Autodesk Inventor part; units mm, degrees
ref_plane "YZ Plane" through (0, 0, 0) normal (1, 0, 0) x (0, 1, 0)
ref_plane "XZ Plane" through (0, 0, 0) normal (0, 1, 0) x (-1, 0, 0)
ref_plane "XY Plane" through (0, 0, 0) normal (0, 0, 1) x (1, 0, 0)
sketch "Sketch1" plane through (0, 0, 0) normal (0, 0, 1) x (1, 0, 0)
  circle A0 centre (0, 0) radius 16.5
  circle A1 centre (15.5, 15.5) radius 1.25
  circle A2 centre (15.5, -15.5) radius 1.55
  circle A3 centre (-15.5, -15.5) radius 1.55
  circle A4 centre (-15.5, 15.5) radius 1.55
  line L0 (-21, 21) -> (21, 21)
  line L1 (21, 21) -> (21, -21)
  line L2 (21, -21) -> (-21, -21)
  line L3 (-21, -21) -> (-21, 21)
  line L4 (-21, 21) -> (21, -21) construction
  line L5 (21, 21) -> (-21, -21) construction
  point P0 (0, 0)
  dimension "d0" = 42
  dimension "d1" = 42
extrude "Extrusion1" add sketch "Sketch1" along normal blind 5
equation "\"BendRadius\" = Thickness"
equation "\"BendReliefWidth\" = Thickness"
equation "\"BendReliefDepth\" = 0.5 * Thickness"
equation "\"CornerReliefSize\" = 4 * Thickness"
equation "\"MinimumRemnant\" = 2 * Thickness"
equation "\"TransitionRadius\" = BendRadius"
equation "\"JacobiRadiusSize\" = Thickness"
equation "\"GapSize\" = Thickness"
properties part number "Motor Mount V2.1"
Here's how the part is built. I have some questions about the finished solid (model axes, mm). Round coordinates to 2 decimals unless told otherwise and drop trailing zeros. Order: outer loops, then holes, each group sorted by start corner. A loop starts at its lowest first (then second) coordinate and runs counter-clockwise, first axis right, second up. Notation, with made-up numbers: (-25.75, 17) -> (29.25, 17) arc R22 cw to (29.25, 23) -> close; hole circle Ø1 at (63, 78.25). An arc over 180 degrees is marked (long way). Use CSV: the item, a comma, the result in double quotes.
1. I want a section at D-D on x = 15.5. List the corners of the cut face in (y, z) for me.
Recorded:
outline,"(-21, 0) -> (-17.05, 0) -> (-17.05, 5) -> (-21, 5) -> close; (-13.95, 0) -> (-5.66, 0) -> (-5.66, 5) -> (-13.95, 5) -> close; (5.66, 0) -> (14.25, 0) -> (14.25, 5) -> (5.66, 5) -> close; (16.75, 0) -> (21, 0) -> (21, 5) -> (16.75, 5) -> close"
2. I want a section at A-A on y = 0. List the corners of the cut face in (x, z) for me, and give its area (3 significant figures).
Recorded:
outline,"(-21, 0) -> (-16.5, 0) -> (-16.5, 5) -> (-21, 5) -> close; (16.5, 0) -> (21, 0) -> (21, 5) -> (16.5, 5) -> close"
area,"45.0 mm2"
3. I want a section at C-C on z = 4.5. List the corners of the cut face in (x, y) for me, and give its area (3 significant figures).
Recorded:
outline,"(-21, -21) -> (21, -21) -> (21, 21) -> (-21, 21) -> close; hole circle Ø3.1 at (-15.5, -15.5); hole circle Ø3.1 at (-15.5, 15.5); hole circle Ø33 at (0, 0); hole circle Ø3.1 at (15.5, -15.5); hole circle Ø2.5 at (15.5, 15.5)"
area,"881 mm2"
4. Thinking about a two-plate mould opening in X: for faces 1 (the face through (15.34, 14.26, 2.46)), 2 (the face through (21, 0, 2)), 3 (the face through (0, -21, 2)), 4 (the face through (-16.64, 14.45, 2.46)), which applies, pulls with the +X half, pulls with the -X half, needs draft (parallel to the pull), parting line crosses it, or undercut?
Recorded:
face 1,"undercut"
face 2,"pulls with the +X half"
face 3,"needs draft"
face 4,"undercut"
5. I need wall thicknesses on line 1 along X through (y, z) = (11, 2.15); line 2 along Y through (x, z) = (-13, 3.1); line 3 along Y through (x, z) = (12, 1.05). Which ranges of each line are inside material? Lowest first, please.
Recorded:
line 1,"x = -21 to -12.3, 12.3 to 21"
line 2,"y = -21 to -10.16, 10.16 to 21"
line 3,"y = -21 to -11.32, 11.32 to 21"
